Part model, mm, in its own coordinate system. A direction names the side the tool comes from. Coordinates: 2 decimals unless noted, no trailing zeros. Loops run counter-clockwise (first coordinate to the right, second up) from the corner with the lowest first, then second, coordinate; pieces in that order, holes last. Notation, with made-up numbers: (77.25, -11) - (110.25, -11) arc R15 ccw to (110.25, 8) - close; hole circle Ø3 at (-11.5, 14). An arc over 180 degrees is marked (long way). Use a Markdown table: item, result. Add a question column.
1) Band-saw the part on C-C (x = 3.25). Give the cut face in (y, z).
2) Probe probe 1 along Y at (x, z) = (4, 0.2); probe 2 along Y at (x, z) = (1, -2.35). List the from-to ranges inside material, lowest first. Write a range as [from, to].
3) Pull direction Z, two halves, no side cores. Call faces 1 (the face through (0.4, 7.366, -1.4)), 2 (the face through (0.57, 7.05, -1.61)), 3 (the face through (2, 3, -3.302)): +Z half, -Z half, draft (parallel to the pull), parting line (faces both ways), or undercut.
4) Band-saw the part on B-B (x = 5.08). Give the cut face in (y, z) (3 decimals), plus the area to 3 significant figures.
5) Band-saw the part on A-A (z = 0). Give the cut face in (x, y) (3 decimals).
6) Tool access for faces 4 (the face through (-0.762, 3, -1)), 5 (the face through (1, 7.1, -1.9)): list every direction of +Z, -Z, +X, -X, +Y, -Y with a clear straight run to the whole face (end or side of a thin tool).
7) Drop flat-ended pins along their axis: P1, Ø1.3, axis at x = 2, z = -1, coming from the -Y side; P2, Ø1, axis at x = 2.5, z = -1.5, coming from the +Y side. Give the stop position or say it passes through.
from build123d import *

# Parameters (mm, degrees)
SKETCH1_W      = 6.35
SKETCH1_H      = 4.318
EXTRUDE1_DEPTH = 6.35
SKETCH2_R      = 0.889
EXTRUDE2_DEPTH = 1.016
EXTRUDE3_DEPTH = 0.635
SKETCH4_R      = 0.2286
EXTRUDE4_DEPTH = 4.7752
SKETCH5_W      = 5.5372
SKETCH5_H      = 2.8702
PCB_TRIM_DEPTH = 11.204353189


with BuildPart() as part:
    # Sketch1 → Extrude1 (new body)
    with BuildSketch(Plane(origin=(0, 0, 0), x_dir=(1, 0, 0), z_dir=(0, 1, 0))):
        with Locations((2.413, 1.143)):
            Rectangle(SKETCH1_W, SKETCH1_H)
    extrude(amount=EXTRUDE1_DEPTH)

    # Sketch2 → Extrude2 (add)
    with BuildSketch(Plane(origin=(0, 6.35, 0), x_dir=(1, 0, 0), z_dir=(0, 1, 0))):
        with Locations(Location((0.762, 1.778, 0), (0, 0, 90))):
            Circle(SKETCH2_R)
    extrude(amount=EXTRUDE2_DEPTH)

    # Sketch3 → Extrude3 (cut)
    with BuildSketch(Plane(origin=(0, 7.366, 0), x_dir=(1, 0, 0), z_dir=(0, 1, 0))):
        Polygon((-0.145336371, 2.326126126), (1.310126126, 0.870663629), (1.669336371, 1.229873874), (0.213873874, 2.685336371), align=None)
    extrude(amount=-EXTRUDE3_DEPTH, mode=Mode.SUBTRACT)

    # Sketch4 → Extrude4 (add)
    with BuildSketch(Plane.XZ):
        with Locations(Location((0, 0, 0), (0, 0, 270))):
            Circle(SKETCH4_R)
        with Locations(Location((5.08, 0, 0), (0, 0, 270))):
            Circle(SKETCH4_R)
        with Locations(Location((2.54, -2.54, 0), (0, 0, 270))):
            Circle(SKETCH4_R)
    extrude(amount=EXTRUDE4_DEPTH)

    # Sketch5 → PCB Trim (cut, through all)
    with BuildSketch(Plane.XY.offset(1.016)):
        with Locations((2.54, -3.3401)):
            Rectangle(SKETCH5_W, SKETCH5_H)
    extrude(amount=-PCB_TRIM_DEPTH, mode=Mode.SUBTRACT)


solid = part.part
Answer block:
| question | item | result |
|---|---|---|
| 1 | outline | (0, -3.3) - (6.35, -3.3) - (6.35, 1.02) - (0, 1.02) - close |
| 2 | probe 1 | [0, 6.35] |
| 2 | probe 2 | [0, 7.37] |
| 3 | face 1 | draft |
| 3 | face 2 | undercut |
| 3 | face 3 | -Z half |
| 4 | outline | (-1.905, -0.229) - (0, -0.229) - (0, -3.302) - (6.35, -3.302) - (6.35, 1.016) - (0, 1.016) - (0, 0.229) - (-1.905, 0.229) - close |
| 4 | area | 28.3 mm2 |
| 5 | outline | (-0.762, 0) - (-0.229, 0) - (-0.229, -1.905) - (0.229, -1.905) - (0.229, 0) - (4.851, 0) - (4.851, -1.905) - (5.309, -1.905) - (5.309, 0) - (5.588, 0) - (5.588, 6.35) - (-0.762, 6.35) - close |
| 6 | face 4 | +Z, -Z, -X, +Y, -Y |
| 6 | face 5 | +Y |
| 7 | P1 | y = 0 |
| 7 | P2 | y = 6.35 |
